Work out the finished part from the listing and answer in its coordinate system (mm). Face numbers are marked on the shaded views. A direction names the side the tool comes from. Coordinates: 2 decimals unless noted, no trailing zeros. Order: outer loops, then holes, each group sorted by start corner. A loop starts at its lowest first (then second) coordinate and runs counter-clockwise, first axis right, second up. Notation, with made-up numbers: (29, -15.5) - (81, -15.5) arc R19 ccw to (81, 16.5) - close; hole circle Ø7 at (-3.75, 45.5). An arc over 180 degrees is marked (long way). Use CSV: the item, a comma, the result in double quotes. Start each with the question number.
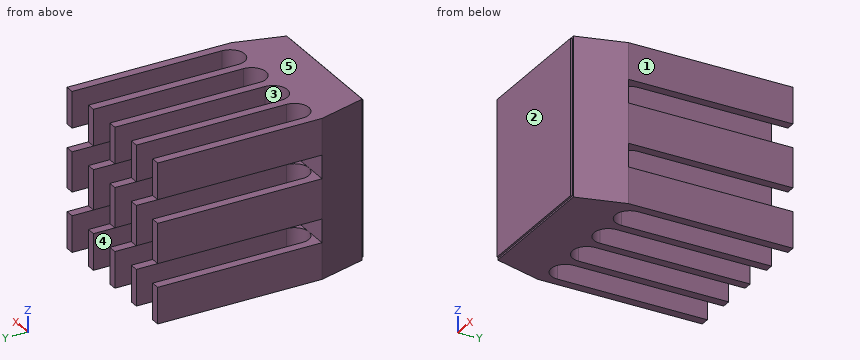
from build123d import *

# Parameters (mm, degrees)
AUFSATZ_LINEAR_AUSTRAGEN1_DEPTH = 4.5
SCHNITT_LINEAR_AUSTRAGEN1_DEPTH = 9
SCHNITT_LINEAR_AUSTRAGEN2_REACH = 17.66
SKIZZE3_W                       = 1.325
SKIZZE3_H                       = 9.3
SKIZZE4_W                       = 7.3
SKIZZE4_H                       = 8.8
AUFSATZ_LINEAR_AUSTRAGEN2_DEPTH = 0.1


with BuildPart() as part:
    # Skizze1 → Aufsatz-Linear austragen1 (new, symmetric)
    with BuildSketch(Plane.XY):
        Polygon((-4.5, 12), (-4.5, 2.7), (-3.75, 0), (3.75, 0), (4.5, 2.7), (4.5, 12), align=None)
    extrude(amount=AUFSATZ_LINEAR_AUSTRAGEN1_DEPTH, both=True)

    # Skizze2 → Schnitt-Linear austragen1 (cut)
    with BuildSketch(Plane.XY.offset(4.5)):
        with BuildLine():
            Line((-2.375, 12), (-2.375, 3.5125))
            ThreePointArc((-2.375, 3.5125), (-3.1875, 2.7), (-4, 3.5125))
            Line((-4, 3.5125), (-4, 12))
            ThreePointArc((-4, 12), (-3.1875, 12.8125), (-2.375, 12))
        make_face()
        with BuildLine():
            Line((-0.25, 12), (-0.25, 3.5125))
            ThreePointArc((-0.25, 3.5125), (-1.0625, 2.7), (-1.875, 3.5125))
            Line((-1.875, 3.5125), (-1.875, 12))
            ThreePointArc((-1.875, 12), (-1.0625, 12.8125), (-0.25, 12))
        make_face()
        with BuildLine():
            Line((1.875, 12), (1.875, 3.5125))
            ThreePointArc((1.875, 3.5125), (1.0625, 2.7), (0.25, 3.5125))
            Line((0.25, 3.5125), (0.25, 12))
            ThreePointArc((0.25, 12), (1.0625, 12.8125), (1.875, 12))
        make_face()
        with BuildLine():
            Line((4, 12), (4, 3.5125))
            ThreePointArc((4, 3.5125), (3.1875, 2.7), (2.375, 3.5125))
            Line((2.375, 3.5125), (2.375, 12))
            ThreePointArc((2.375, 12), (3.1875, 12.8125), (4, 12))
        make_face()
    extrude(amount=-SCHNITT_LINEAR_AUSTRAGEN1_DEPTH, mode=Mode.SUBTRACT)

    # Schnitt-Linear austragen2: up to this face of the body (flat: up to its plane)
    schnitt_linear_austragen2_end = Plane(part.part.faces().sort_by_distance((-4.5, 7.35, 0))[0])
    # Skizze3 → Schnitt-Linear austragen2 (cut, up to the picked face)
    with BuildSketch(Plane(origin=(4.5, 0, 0), x_dir=(0, 0, -1), z_dir=(1, 0, 0)), mode=Mode.PRIVATE) as schnitt_linear_austragen2_sk1:
        with Locations((-1.7875, 7.35)):
            Rectangle(SKIZZE3_W, SKIZZE3_H)
    schnitt_linear_austragen2_tool1 = split(extrude(schnitt_linear_austragen2_sk1.sketch, amount=-SCHNITT_LINEAR_AUSTRAGEN2_REACH, mode=Mode.PRIVATE), bisect_by=schnitt_linear_austragen2_end, keep=Keep.BOTH, mode=Mode.PRIVATE)
    # Skizze3 → Schnitt-Linear austragen2 (cut, up to the picked face)
    with BuildSketch(Plane(origin=(4.5, 0, 0), x_dir=(0, 0, -1), z_dir=(1, 0, 0)), mode=Mode.PRIVATE) as schnitt_linear_austragen2_sk2:
        with Locations((1.7875, 7.35)):
            Rectangle(SKIZZE3_W, SKIZZE3_H)
    schnitt_linear_austragen2_tool2 = split(extrude(schnitt_linear_austragen2_sk2.sketch, amount=-SCHNITT_LINEAR_AUSTRAGEN2_REACH, mode=Mode.PRIVATE), bisect_by=schnitt_linear_austragen2_end, keep=Keep.BOTH, mode=Mode.PRIVATE)
    add(schnitt_linear_austragen2_tool1.solids().sort_by(Axis((4.5, 7.35, 1.7875), (-1, 0, 0)))[0], mode=Mode.SUBTRACT)
    add(schnitt_linear_austragen2_tool2.solids().sort_by(Axis((4.5, 7.35, -1.7875), (-1, 0, 0)))[0], mode=Mode.SUBTRACT)

    # Skizze4 → Aufsatz-Linear austragen2 (add)
    with BuildSketch(Plane.XZ):
        Rectangle(SKIZZE4_W, SKIZZE4_H)
    extrude(amount=AUFSATZ_LINEAR_AUSTRAGEN2_DEPTH)


solid = part.part
1) A flat-ended cylindrical pin translates along its axis: P1, Ø1.1, axis at x = -2.5, y = 6.5, coming from the -Z side. Find the tip coordinate at first contact, or state that the pin passes through.
2) For a pull along X with two mould halves and no side action, classify the marked faces 1, 2 and 3 as +X half, -X half, draft (parallel to the pull), parting line (faces both ways), or undercut.
3) For the marked faces 4 and 5, determine the directions among +Z, -Z, +X, -X, +Y, -Y from which every point of the face is accessible in a straight line to the end or side of a thin tool.
4) The part is cut by section C-C on y = 8.25. State how many separate pieces and enclosed holes the cut face has, plus the area to 3 significant figures.
5) The part is cut by section B-B on x = 0. Determine the outline of the cut face in (y, z) (3 decimals).
6) The part is cut by section A-A on z = -1.5. Determine the outline of the cut face in (x, y).
7) Straight lines are drawn through the part: line 1 (X direction, y = 4.5, z = -0.5) (3 decimals); line 2 (Z direction, x = 2, y = 11) (3 decimals); line 3 (Y direction, x = 1.25, z = -2). For each, find the intervals that lie inside material, in ascending order. Write a range as [from, to].
Answer key:
1,P1,"z = -4.5"
2,face 1,"+X half"
2,face 2,"draft"
2,face 3,"undercut"
3,face 4,"+Z, -Z, +Y"
3,face 5,"+Z, +X, -X, +Y, -Y"
4,separate pieces,"15"
4,enclosed holes,"0"
4,area,"15.9 mm^2"
5,outline,"(-0.1, -4.4) - (0, -4.4) - (0, -4.5) - (12, -4.5) - (12, -2.45) - (2.7, -2.45) - (2.7, -1.125) - (12, -1.125) - (12, 1.125) - (2.7, 1.125) - (2.7, 2.45) - (12, 2.45) - (12, 4.5) - (0, 4.5) - (0, 4.4) - (-0.1, 4.4) - close"
6,outline,"(-4.5, 2.7) - (-3.75, 0) - (-3.65, 0) - (-3.65, -0.1) - (3.65, -0.1) - (3.65, 0) - (3.75, 0) - (4.5, 2.7) - close"
7,line 1,"[-4.5, -4], [-2.375, -1.875], [-0.25, 0.25], [1.875, 2.375], [4, 4.5]"
7,line 2,"[-4.5, -2.45], [-1.125, 1.125], [2.45, 4.5]"
7,line 3,"[-0.1, 2.7]"
